Read the model definition and answer for the solid it produces. Units are mm, in the model's axes. Face numbers are marked on the shaded views. Coordinates: 2 decimals unless noted, no trailing zeros. Write each loop counter-clockwise with the first axis right and the second up, starting at its lowest first coordinate (ties: lowest second). Pieces come first, ordered by that corner, then holes. Notation, with made-up numbers: (2, 70.5) - (61, 70.5) arc R28 ccw to (61, 93.5) - close; hole circle Ø6 at (40, -39.75). An arc over 180 degrees is marked (long way). Use a Markdown table: item, result.
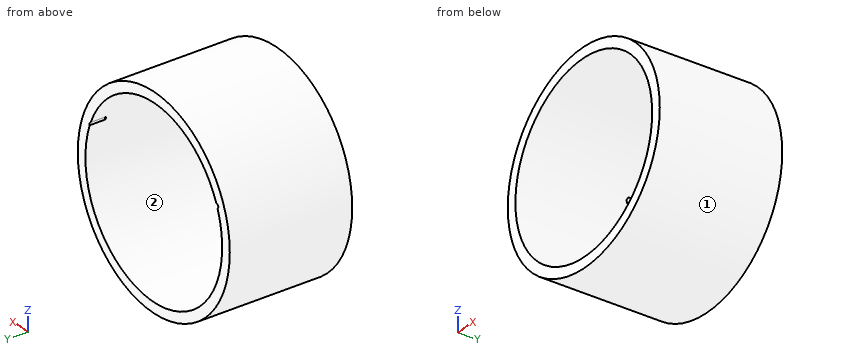
from build123d import *

# Parameters (mm, degrees)
SKETCH1_R             = 50
BOSS_EXTRUDE1_DEPTH   = 60
SKETCH2_R             = 45
CUT_EXTRUDE1_DEPTH    = 93.736184955
M3_TAPPED_HOLE2_D     = 2.5
M3_TAPPED_HOLE2_DEPTH = 7.5
M3_TAPPED_HOLE2_TIP   = 0.751075774


with BuildPart() as part:
    # Sketch1 → Boss-Extrude1 (new body)
    with BuildSketch(Plane(origin=(0, 0, 0), x_dir=(1, 0, 0), z_dir=(0, 1, 0))):
        with Locations(Location((0, 0, 0), (0, 0, 270))):
            Circle(SKETCH1_R)
    extrude(amount=BOSS_EXTRUDE1_DEPTH)

    # Sketch2 → Cut-Extrude1 (cut, through all)
    with BuildSketch(Plane(origin=(0, 60, 0), x_dir=(1, 0, 0), z_dir=(0, 1, 0))):
        with Locations(Location((0, 0, 0), (0, 0, 270))):
            Circle(SKETCH2_R)
    extrude(amount=-CUT_EXTRUDE1_DEPTH, mode=Mode.SUBTRACT)

    # M3 Tapped Hole2
    with Locations(Plane(origin=(-125, 60, -260), x_dir=(-1, 0, 0), z_dir=(0, 1, 0))):
        with Locations((-125.588729382, 346.343542242), (-83.789316087, 277.051897383), (-165.985477802, 276.210298458), (165.689643288, 275.872555658), (83.529497195, 276.252926704), (125.273893117, 347.014910337)):
            Hole(M3_TAPPED_HOLE2_D / 2, depth=M3_TAPPED_HOLE2_DEPTH)
            with Locations((0, 0, -(M3_TAPPED_HOLE2_DEPTH + M3_TAPPED_HOLE2_TIP / 2))):  # 118° drill point
                Cone(0, M3_TAPPED_HOLE2_D / 2, M3_TAPPED_HOLE2_TIP, mode=Mode.SUBTRACT)


solid = part.part
(1) A cutting plane is placed at C-C, the plane y = 5. Write down the section's boundary in (x, z).
Report:
| item | result |
|---|---|
| outline | circle Ø100 at (0, 0); hole circle Ø90 at (0, 0) |
(2) The mould has two halves that part along Z. Classify the marked faces 1 and 2: pulls with the +Z half, pulls with the -Z half, needs draft (parallel to the pull), parting line crosses it, or undercut.
Report:
| item | result |
|---|---|
| face 1 | parting line crosses it |
| face 2 | undercut |
(3) Each of these flat-tipped pins is pushed along its axis until it touches: P1, Ø10, axis at y = 50.5, z = 23.5, coming from the -X side; P2, Ø8, axis at x = -33.5, y = 26.5, coming from the +Z side; P3, Ø8, axis at y = 11.5, z = 4.5, coming from the -X side. Where does it stop, or does it pass through?
Report:
| item | result |
|---|---|
| P1 | stops at x = -46.45 |
| P2 | stops at z = 40.37 |
| P3 | stops at x = -50 |
(4) Straight lines are drawn through the part: L1, parallel to X at y = 33, z = 0; L2, parallel to Z at x = -3, y = 36.5; L3, parallel to Z at x = -14, y = 15. For each, find the intervals that lie inside material, in ascending order.
Report:
| item | result |
|---|---|
| L1 | x = -50 to -45, 45 to 50 |
| L2 | z = -49.91 to -44.9, 44.9 to 49.91 |
| L3 | z = -48 to -42.77, 42.77 to 48 |
(5) A cutting plane is placed at B-B, the plane x = 0. Write down the section's boundary in (y, z), and give its area (3 significant figures).
Report:
| item | result |
|---|---|
| outline | (0, -50) - (60, -50) - (60, -45) - (0, -45) - close; (0, 45) - (60, 45) - (60, 50) - (0, 50) - close |
| area | 600 mm² |
(6) A cutting plane is placed at A-A, the plane z = 0. Write down the section's boundary in (x, y).
Report:
| item | result |
|---|---|
| outline | (-50, 0) - (-45, 0) - (-45, 60) - (-50, 60) - close; (45, 0) - (50, 0) - (50, 60) - (45, 60) - close |
